Autodesk Inventor part; units mm, degrees
ref_plane "Work Plane1" through (-304.8, 152.4, 3.175) normal (0, 1, 0) x (1, 0, 0)
ref_plane "YZ Plane" through (0, 0, 0) normal (1, 0, 0) x (0, 1, 0)
ref_plane "XZ Plane" through (0, 0, 0) normal (0, 1, 0) x (-1, 0, 0)
sketch "Sketch1" plane through (0, 0, 0) normal (0, 0, 1) x (1, 0, 0)
  line L0 (-426.72, 0) -> (426.72, 0)
  line L1 (0, -417.83) -> (0, 417.83)
  line L2 (-304.8, 298.45) -> (304.8, 298.45)
  line L3 (304.8, 298.45) -> (304.8, -298.45)
  line L4 (304.8, -298.45) -> (-304.8, -298.45)
  line L5 (-304.8, -298.45) -> (-304.8, 298.45)
  point P0 (0, 0)
  point P1 (-304.8, 0)
  point P2 (0, 298.45)
  dimension "d0" = 609.6
  dimension "d1" = 596.9
extrude "Base" add sketch "Sketch1" along normal mid plane 6.35
sketch "Sketch2" plane through (0, 0, 3.175) normal (0, 0, 1) x (1, 0, 0)
  line L0 (304.8, -298.45) -> (-304.8, -298.45)
  line L1 (-196.85, -298.45) -> (-196.85, 6.35)
  line L2 (-196.85, 6.35) -> (196.85, 6.35)
  line L3 (196.85, 6.35) -> (196.85, -298.45)
  point P0 (0, 0)
  point P1 (0, 6.35)
  dimension "d4" = 304.8
  dimension "d5" = 393.7
extrude "Extrusion2" cut sketch "Sketch2" against normal through all
ref_plane "Work Plane1" through (-304.8, 152.4, 3.175) normal (0, 1, 0) x (1, 0, 0)
properties part number "electrical board seal front" material "ABS Plastic"
Input: part model. Units: mm. Frame: model coordinates. Coordinates: 2 decimals unless noted, no trailing zeros. Order: outer loops, then holes, each group sorted by start corner. A loop starts at its lowest first (then second) coordinate and runs counter-clockwise, first axis right, second up. Notation, with made-up numbers: M 23.5,80.25 L 61.5,80.25 A22 ccw 61.5,100.25 Z; hole C 35.25,-18 d8. An arc over 180 degrees is marked long. Write item = value, one per line. Start each with the question number.
(1) Section C-C on x = 2. Output: boundary loops of the cut face in (y, z) (3 decimals), and give its area (3 significant figures).
(2) Line query: line 1 along X through (y, z) = (-24.5, -2.5); line 2 along Y through (x, z) = (183, 2.25). Output: solid intervals per line, ascending. Write a range as [from, to].
(3) Section A-A on y = -249.5. Output: boundary loops of the cut face in (x, z) (3 decimals).
(4) First-contact query: P1, Ø3, axis at x = 67, z = 0, coming from the -Y side. Flat tip, straight axial feed; report the tip coordinate or a pass-through.
(5) Section B-B on z = -0.5. Output: boundary loops of the cut face in (x, y), and give its area (3 significant figures).
Result set:
q1.outline = M 6.35,-3.175 L 298.45,-3.175 L 298.45,3.175 L 6.35,3.175 Z
q1.area = 1,850 mm²
q2.line_1 = [-304.8, -196.85], [196.85, 304.8]
q2.line_2 = [6.35, 298.45]
q3.outline = M -304.8,-3.175 L -196.85,-3.175 L -196.85,3.175 L -304.8,3.175 Z; M 196.85,-3.175 L 304.8,-3.175 L 304.8,3.175 L 196.85,3.175 Z
q4.P1 = 6.35
q5.outline = M -304.8,-298.45 L -196.85,-298.45 L -196.85,6.35 L 196.85,6.35 L 196.85,-298.45 L 304.8,-298.45 L 304.8,298.45 L -304.8,298.45 Z
q5.area = 244,000 mm²
